Geometry check sheet. Reference: the model listing, model coordinates, mm. Face numbers are marked on the shaded views. A direction names the side the tool comes from. Round coordinates to 2 decimals unless told otherwise and drop trailing zeros. Order: outer loops, then holes, each group sorted by start corner. A loop starts at its lowest first (then second) coordinate and runs counter-clockwise, first axis right, second up.
```python
from build123d import *

# Parameters (mm, degrees)
F0_W     = 35.56
F0_H     = 35.56
F1_DEPTH = 5.08
F2_W     = 19.812
F2_H     = 4.572
F3_DEPTH = 2.54
F4_W     = 19.812
F4_H     = 4.572
F5_DEPTH = 2.54
F6_W     = 20.32
F6_H     = 5.08
F7_DEPTH = 2.54
F8_W     = 20.32
F8_H     = 5.08
F9_DEPTH = 2.54


with BuildPart() as f1:
    # F0 (on Top) → F1 (new body, symmetric)
    with BuildSketch(Plane.XY):
        Rectangle(F0_W, F0_H)
        Polygon((8.6485677083, -8.2902777778), (8.6485677083, -12.7), (-10.0927517361, -12.7), (-10.0927517361, -9.2383680556), (1.984375, 8.0753038194), (-9.7620225694, 8.0753038194), (-9.7620225694, 12.4850260417), (8.3233506944, 12.4850260417), (8.3233506944, 9.0399305556), (-3.7372395833, -8.2902777778), align=None, mode=Mode.SUBTRACT)
    extrude(amount=F1_DEPTH, both=True)

    # F2 (on face) → F3 (join)
    with BuildSketch(Plane(origin=(0, 17.78, 0), x_dir=(-1, 0, 0), z_dir=(0, 1, 0))):
        Rectangle(F2_W, F2_H)
    extrude(amount=F3_DEPTH)

    # F4 (on face) → F5 (join)
    with BuildSketch(Plane(origin=(-17.78, 0, 0), x_dir=(0, -1, 0), z_dir=(-1, 0, 0))):
        Rectangle(F4_W, F4_H)
    extrude(amount=F5_DEPTH)

    # F6 (on face) → F7 (cut)
    with BuildSketch(Plane.XZ.offset(17.78)):
        Rectangle(F6_W, F6_H)
    extrude(amount=-F7_DEPTH, mode=Mode.SUBTRACT)

    # F8 (on face) → F9 (cut)
    with BuildSketch(Plane.YZ.offset(17.78)):
        Rectangle(F8_W, F8_H)
    extrude(amount=-F9_DEPTH, mode=Mode.SUBTRACT)


solid = f1.part
```
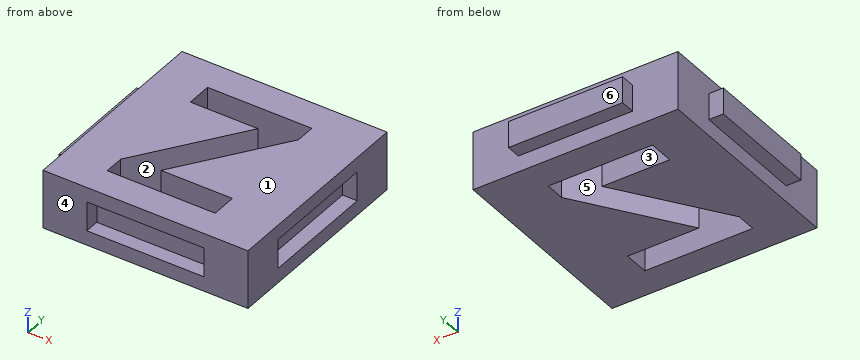
(1) Draft check along Y on the marked faces 1, 2, 3 and 4. Enter one of: released by +Y, released by -Y, zero draft, split by the parting line, or undercut.
Returned:
face 1: zero draft
face 2: undercut
face 3: undercut
face 4: released by -Y
(2) Depth check by flat-ended pin: P1, Ø3, axis at x = -19.5, z = -0.5, coming from the +Y side; P2, Ø1.3, axis at y = -16, z = 0, coming from the -X side; P3, Ø3, axis at x = 16.5, z = -1, coming from the +Y side. Enter the tip coordinate at first touch or a pass-through.
Returned:
P1: stops at y = 9.91
P2: stops at x = -17.78
P3: stops at y = 17.78
(3) Sectioned sample at B-B, the plane y = -12. Record the cut outline in (x, z).
Returned:
outline: (-17.78, -5.08) - (-10.09, -5.08) - (-10.09, 5.08) - (-17.78, 5.08) - close; (8.65, -5.08) - (17.78, -5.08) - (17.78, 5.08) - (8.65, 5.08) - close
(4) Set-up check for the marked faces 5 and 6: record each of +Z, -Z, +X, -X, +Y, -Y from which the full face is reachable in a straight line by a thin tool's end or side.
Returned:
face 5: +Z, -Z
face 6: +Z, -Z, +X, -X, +Y
(5) Sectioned sample at D-D, the plane z = -3.75. Record the cut outline in (x, y).
Returned:
outline: (-17.78, -17.78) - (17.78, -17.78) - (17.78, 17.78) - (-17.78, 17.78) - close; hole (-10.09, -12.7) - (8.65, -12.7) - (8.65, -8.29) - (-3.74, -8.29) - (8.32, 9.04) - (8.32, 12.49) - (-9.76, 12.49) - (-9.76, 8.08) - (1.98, 8.08) - (-10.09, -9.24) - close
(6) Material ranges on line 1 (X direction, y = 10.5, z = -1.5); line 2 (Y direction, x = 16.5, z = -0.25); line 3 (Y direction, x = -5, z = -3.75), recorded low to high.
Returned:
line 1: x = -17.78 to -9.76, 8.32 to 17.78
line 2: y = -17.78 to -10.16, 10.16 to 17.78
line 3: y = -17.78 to -12.7, -1.94 to 8.08, 12.49 to 17.78
(7) Sectioned sample at C-C, the plane x = -9. Record the cut outline in (y, z), and give its area (3 significant figures).
Returned:
outline: (-17.78, -5.08) - (-12.7, -5.08) - (-12.7, 5.08) - (-17.78, 5.08) - (-17.78, 2.54) - (-15.24, 2.54) - (-15.24, -2.54) - (-17.78, -2.54) - close; (-7.67, -5.08) - (8.08, -5.08) - (8.08, 5.08) - (-7.67, 5.08) - close; (12.49, -5.08) - (17.78, -5.08) - (17.78, -2.29) - (20.32, -2.29) - (20.32, 2.29) - (17.78, 2.29) - (17.78, 5.08) - (12.49, 5.08) - close
area: 264 mm2
